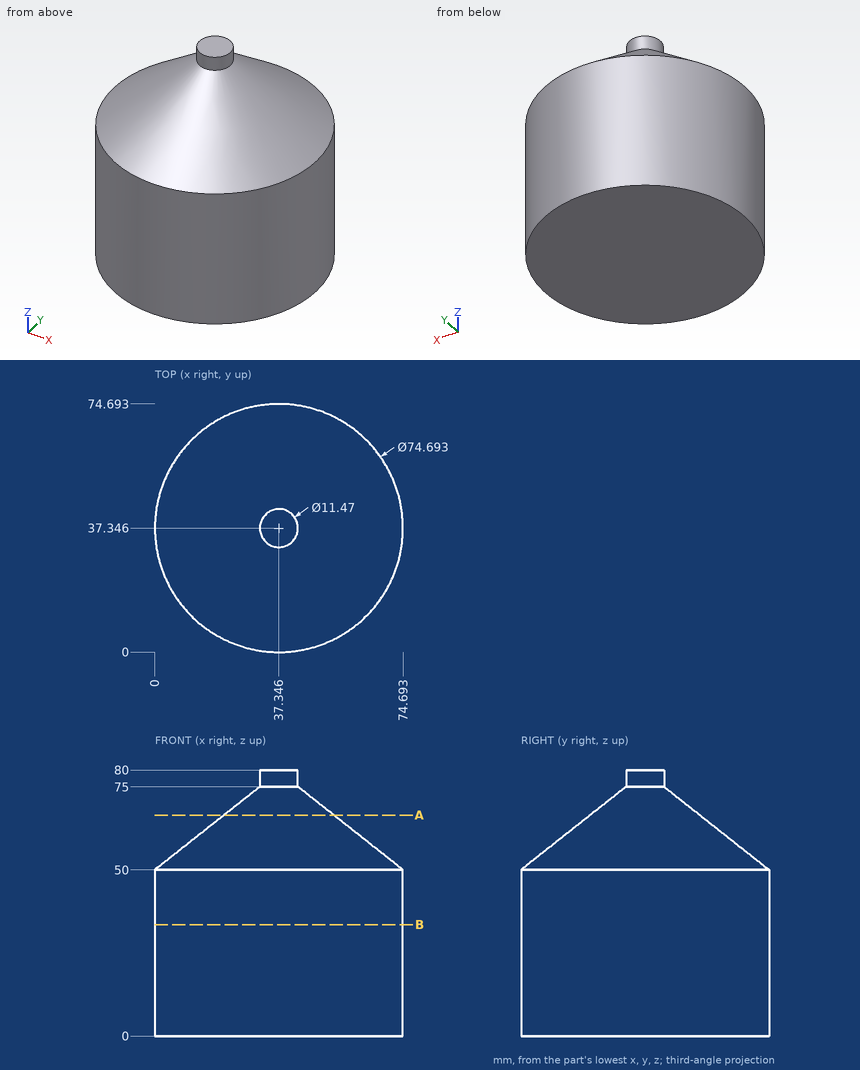
Design review of the part shown in the three views and the two pictorial views. Dimensions are in mm from the part's minimum x, y and z. Round coordinates to 2 decimals unless told otherwise and drop trailing zeros. Order: outer loops, then holes, each group sorted by start corner. A loop starts at its lowest first (then second) coordinate and runs counter-clockwise, first axis right, second up.
Item 1: Add section B-B, the plane z = 33.5. State the section outline as (x, y) points.
Working result:
outline: circle Ø74.69 at (37.35, 37.35)
Item 2: Add section A-A, the plane z = 66.5. State the section outline as (x, y) points (1 decimal).
Working result:
outline: circle Ø33 at (37.3, 37.3)
Item 3: For pin 1 (10 mm diameter, centred on y = 50, z = 38.5, fed in from -X); pin 2 (12 mm diameter, centred on x = 44, y = 20.5, fed in from +Z) (1 decimal); pin 3 (6 mm diameter, centred on y = 59, z = 29.5, fed in from -X); pin 4 (2 mm diameter, centred on x = 67, z = 59, fed in from +Y), all flat-tipped, find the tip position at first contact; note any pin that passes through.
Working result:
pin 1: stops at x = 0.79
pin 2: stops at z = 70
pin 3: stops at x = 4.99
pin 4: passes through
Item 4: To check wall thickness, follow probe 1 along Z at (x, y) = (35, 26.5); probe 2 along Z at (x, y) = (33, 11); probe 3 along X at (y, z) = (38, 4.5) (1 decimal). State the ranges of each line that lie inside material, in increasing order.
Working result:
probe 1: z = 0 to 70.76
probe 2: z = 0 to 58.42
probe 3: x = 0 to 74.7
